Autodesk Inventor part; units mm, degrees
ref_plane "YZ Plane" through (0, 0, 0) normal (1, 0, 0) x (0, 1, 0)
ref_plane "XZ Plane" through (0, 0, 0) normal (0, 1, 0) x (-1, 0, 0)
ref_plane "XY Plane" through (0, 0, 0) normal (0, 0, 1) x (1, 0, 0)
sketch "Sketch1" plane through (0, 0, 0) normal (0, 0, 1) x (1, 0, 0)
  line L0 (0, 0) -> (16, 0)
  line L1 (16, 0) -> (16, 8)
  line L2 (16, 8) -> (8, 8)
  line L3 (8, 8) -> (8, 16)
  line L4 (8, 16) -> (0, 16)
  line L5 (0, 16) -> (0, 0)
  dimension "d0" = 16
  dimension "d1" = 16
  dimension "d2" = 8
  dimension "d3" = 8
extrude "Extrusion1" add sketch "Sketch1" along normal blind 9.6
sketch "Sketch2" plane through (0, 0, 9.6) normal (0, 0, 1) x (1, 0, 0)
  line L0 (16, 8) -> (16, 0)
  line L1 (8, 8) -> (16, 8)
  line L2 (8, 16) -> (8, 8)
  line L3 (0, 16) -> (8, 16)
  circle A0 centre (4, 12) radius 2.5
  circle A1 centre (4, 4) radius 2.5
  circle A2 centre (12, 4) radius 2.5
  point P0 (4, 16)
  point P1 (16, 4)
  point P2 (8, 12)
  point P3 (12, 8)
  dimension "d6" = 5
extrude "Extrusion2" add sketch "Sketch2" along normal blind 1.6
shell "Shell1" thickness 1.5 removed faces 1 at (2.6667, 8, 0)
equation "\"d0\" = d1"
equation "\"d2\" = 0.5 * d1"
equation "\"d3\" = d2"
properties part number "2357" material "Steel"
The model under review builds one solid part; all positions refer to its coordinate system, in mm. A direction names the side the tool comes from. Round coordinates to 2 decimals unless told otherwise and drop trailing zeros. Loops run counter-clockwise (first coordinate to the right, second up) from the corner with the lowest first, then second, coordinate; pieces in that order, holes last. Notation, with made-up numbers: (-16, 6) - (25, 6) arc R21 cw to (25, 38) - close; hole circle Ø10 at (-20.5, 85). An arc over 180 degrees is marked (long way). Use CSV: the item, a comma, the result in double quotes.
(1) Take a section at D-D, the plane y = 8.75. Give the boundary of the cut face in (x, z), plus the area to 3 significant figures.
Working result:
outline,"(0, 0) - (1.5, 0) - (1.5, 8.1) - (6.5, 8.1) - (6.5, 0) - (8, 0) - (8, 9.6) - (0, 9.6) - close"
area,"36.3 mm^2"
(2) Clearance check with flat-ended pins moving along their axes: P1, Ø3, axis at x = 10.5, y = 14, coming from the -Z side; P2, Ø2.5, axis at y = 11.5, z = 3, coming from the +X side; P3, Ø2, axis at x = 14, z = 2, coming from the +Y side; P4, Ø1.2, axis at x = 4, y = 4, coming from the -Z side. State where each tip first meets the part, or that it passes through.
Working result:
P1,"passes through"
P2,"stops at x = 8"
P3,"stops at y = 8"
P4,"stops at z = 9.7"
(3) The part is to be moulded in two halves that separate along X. For faces 4 (the flat face through (1.5, 8, 4)), 5 (the flat face through (0, 8, 5)), 6 (the flat face through (4, 4, 11.2)), say which applies: pulls with the +X half, pulls with the -X half, needs draft (parallel to the pull), parting line crosses it, or undercut.
Working result:
face 4,"undercut"
face 5,"pulls with the -X half"
face 6,"needs draft"
(4) Machinability: for faces 1 (the flat face through (8, 12, 5)), 2 (the flat face through (4, 14.5, 4)), 3 (the cylindrical face through (9.5, 3.9, 10.4)), which of the approach directions +Z, -Z, +X, -X, +Y, -Y give a long, thin tool a straight path to every point of the face, cutting with its end or side? Answer none if there is none.
Working result:
face 1,"+Z, -Z, +X, +Y"
face 2,"-Z"
face 3,"+Z"
(5) Take a section at B-B, the plane x = 12. Give the boundary of the cut face in (y, z).
Working result:
outline,"(0, 0) - (1.5, 0) - (1.5, 8.1) - (3, 8.1) - (3, 9.7) - (5, 9.7) - (5, 8.1) - (6.5, 8.1) - (6.5, 0) - (8, 0) - (8, 9.6) - (6.5, 9.6) - (6.5, 11.2) - (1.5, 11.2) - (1.5, 9.6) - (0, 9.6) - close"
(6) Take a section at C-C, the plane z = 3.25. Give the boundary of the cut face in (x, y), plus the area to 3 significant figures.
Working result:
outline,"(0, 0) - (16, 0) - (16, 8) - (8, 8) - (8, 16) - (0, 16) - close; hole (1.5, 1.5) - (14.5, 1.5) - (14.5, 6.5) - (6.5, 6.5) - (6.5, 14.5) - (1.5, 14.5) - close"
area,"87.0 mm^2"
(7) For line 1 (X direction, y = 4, z = 9.1); line 2 (Y direction, x = 5.5, z = 1), list the stretches that pass through material, from the lowest coordinate up.
Working result:
line 1,"x = 0 to 3, 5 to 11, 13 to 16"
line 2,"y = 0 to 1.5, 14.5 to 16"
(8) Take a section at A-A, the plane y = 4. Give the boundary of the cut face in (x, z).
Working result:
outline,"(0, 0) - (1.5, 0) - (1.5, 8.1) - (3, 8.1) - (3, 9.7) - (5, 9.7) - (5, 8.1) - (11, 8.1) - (11, 9.7) - (13, 9.7) - (13, 8.1) - (14.5, 8.1) - (14.5, 0) - (16, 0) - (16, 9.6) - (14.5, 9.6) - (14.5, 11.2) - (9.5, 11.2) - (9.5, 9.6) - (6.5, 9.6) - (6.5, 11.2) - (1.5, 11.2) - (1.5, 9.6) - (0, 9.6) - close"
